```python
from build123d import *

# Parameters (mm, degrees)
BOSS_EXTRUDE1_DEPTH     = 6.35
SKETCH2_W               = 38.1
SKETCH2_H               = 6.35
CUT_EXTRUDE1_DEPTH      = 6.35
CUT_EXTRUDE1_DEPTH_BACK = 13.97


with BuildPart() as part:
    # Sketch1 → Boss-Extrude1 (new body)
    with BuildSketch(Plane(origin=(0, 0, 0), x_dir=(1, 0, 0), z_dir=(0, 1, 0))):
        Polygon((-63.5, -79.375), (63.5, -79.375), (63.5, -22.225), (69.85, -22.225), (69.85, 28.575), (63.5, 28.575), (63.5, 79.375), (-63.5, 79.375), (-63.5, 28.575), (-69.85, 28.575), (-69.85, -22.225), (-63.5, -22.225), align=None)
    extrude(amount=BOSS_EXTRUDE1_DEPTH)

    # Sketch2 → Cut-Extrude1 (cut, two sides)
    with BuildSketch(Plane(origin=(0, 6.35, 0), x_dir=(1, 0, 0), z_dir=(0, 1, 0))) as cut_extrude1_sk:
        with Locations((-44.45, -76.2)):
            Rectangle(SKETCH2_W, SKETCH2_H)
        with Locations((44.45, -76.2)):
            Rectangle(SKETCH2_W, SKETCH2_H)
    extrude(amount=CUT_EXTRUDE1_DEPTH, mode=Mode.SUBTRACT)
    extrude(cut_extrude1_sk.sketch, amount=-CUT_EXTRUDE1_DEPTH_BACK, mode=Mode.SUBTRACT)


solid = part.part
```
Check sheet for the modelled part. Datum: model origin and axes. Units: mm. A direction names the side the tool comes from. Round coordinates to 2 decimals unless told otherwise and drop trailing zeros. Loops run counter-clockwise (first coordinate to the right, second up) from the corner with the lowest first, then second, coordinate; pieces in that order, holes last. Notation, with made-up numbers: (82.25, 62) - (90.25, 62) arc R13 cw to (90.25, 77) - close; hole circle Ø8 at (-29, -4.5). An arc over 180 degrees is marked (long way). Write item = value, one per line. Start each with the question number.
Q1. Section check B-B (x = 40). Record the boundary of the cut face in (y, z) (3 decimals).
Q2. Section check A-A (y = 1.75). Record the boundary of the cut face in (x, z) (3 decimals), plus the area to 3 significant figures.
Q3. Section check C-C (z = -41.5). Record the boundary of the cut face in (x, y), plus the area to 3 significant figures.
Q4. Access from +Z, -Z, +X, -X, +Y, -Y to the whole of each face (thin tool, end or side, straight path). Record for faces 1 (the face through (-63.5, 3, -54)), 2 (the face through (63.5, 3, -54)), 3 (the face through (-1, 0, -1)), 4 (the face through (25.4, 3, 76)), 5 (the face through (-67, 3, 22.225)).
Q5. Thickness scan on L1, parallel to Z at x = 25.5, y = 4 (3 decimals); L2, parallel to X at y = 6.25, z = -60.5; L3, parallel to X at y = 4.5, z = 73.5. Record the ranges inside material, lowest first.
Q6. Depth check by flat-ended pin: P1, Ø1.9, axis at y = 3.5, z = 75, coming from the -X side; P2, Ø3, axis at y = 2.5, z = 45, coming from the +X side; P3, Ø1.9, axis at x = 36, y = 2, coming from the +Z side (3 decimals). Enter the tip coordinate at first touch or a pass-through.
Derived:
q1.outline = (0, -79.375) - (6.35, -79.375) - (6.35, 73.025) - (0, 73.025) - close
q2.outline = (-69.85, -28.575) - (-63.5, -28.575) - (-63.5, -79.375) - (63.5, -79.375) - (63.5, -28.575) - (69.85, -28.575) - (69.85, 22.225) - (63.5, 22.225) - (63.5, 73.025) - (25.4, 73.025) - (25.4, 79.375) - (-25.4, 79.375) - (-25.4, 73.025) - (-63.5, 73.025) - (-63.5, 22.225) - (-69.85, 22.225) - close
q2.area = 20,300 mm^2
q3.outline = (-63.5, 0) - (63.5, 0) - (63.5, 6.35) - (-63.5, 6.35) - close
q3.area = 806 mm^2
q4.face_1 = -Z, -X, +Y, -Y
q4.face_2 = -Z, +X, +Y, -Y
q4.face_3 = +Z, -Z, +X, -X, -Y
q4.face_4 = +Z, +X, +Y, -Y
q4.face_5 = +Z, -X, +Y, -Y
q5.L1 = -79.375 to 73.025
q5.L2 = -63.5 to 63.5
q5.L3 = -25.4 to 25.4
q6.P1 = -25.4
q6.P2 = 63.5
q6.P3 = 73.025
